from build123d import *

# Parameters (mm, degrees)
SKETCH1_W            = 604
SKETCH1_H            = 470
BOSS_EXTRUDE1_DEPTH  = 3
FILLET1_R            = 3
M5_CLEARANCE_HOLE1_D = 5.5
CUT_EXTRUDE5_DEPTH   = 766.326727614
SKETCH10_W           = 50
SKETCH10_H           = 80
CUT_EXTRUDE6_DEPTH   = 766.326727614
FILLET5_R            = 3


with BuildPart() as part:
    # Sketch1 → Boss-Extrude1 (new body)
    with BuildSketch(Plane.XY):
        with Locations((302, 235)):
            Rectangle(SKETCH1_W, SKETCH1_H)
    extrude(amount=BOSS_EXTRUDE1_DEPTH)

    # Fillet1
    fillet1_edges = [part.edges().sort_by_distance(p)[0] for p in [
        (0, 470, 1.5),
        (604, 470, 1.5),
        (604, 0, 1.5),
        (0, 0, 1.5),
    ]]
    fillet(fillet1_edges, radius=FILLET1_R)

    # M5 Clearance Hole1 (through all)
    with Locations(Plane(origin=(0, 0, 0), x_dir=(-1, 0, 0), z_dir=(0, 0, -1))):
        with Locations((-594, 460), (-394, 460), (-210, 460), (-10, 460), (-10, 10), (-210, 10), (-394, 10), (-594, 10), (-544, 410), (-544, 60), (-35, 410), (-35, 60), (-109.625, 410), (-109.625, 60)):
            Hole(M5_CLEARANCE_HOLE1_D / 2)

    # Sketch9 → Cut-Extrude5 (cut, through all)
    with BuildSketch(Plane.XY.offset(3)):
        with BuildLine():
            Line((32, 412.75), (38, 412.75))
            ThreePointArc((38, 412.75), (40.75, 410), (38, 407.25))
            Line((38, 407.25), (32, 407.25))
            ThreePointArc((32, 407.25), (29.25, 410), (32, 412.75))
        make_face()
        with BuildLine():
            Line((106.625, 412.75), (112.625, 412.75))
            ThreePointArc((112.625, 412.75), (115.375, 410), (112.625, 407.25))
            Line((112.625, 407.25), (106.625, 407.25))
            ThreePointArc((106.625, 407.25), (103.875, 410), (106.625, 412.75))
        make_face()
        with BuildLine():
            Line((32, 62.75), (38, 62.75))
            ThreePointArc((38, 62.75), (40.75, 60), (38, 57.25))
            Line((38, 57.25), (32, 57.25))
            ThreePointArc((32, 57.25), (29.25, 60), (32, 62.75))
        make_face()
        with BuildLine():
            Line((106.625, 62.75), (112.625, 62.75))
            ThreePointArc((112.625, 62.75), (115.375, 60), (112.625, 57.25))
            Line((112.625, 57.25), (106.625, 57.25))
            ThreePointArc((106.625, 57.25), (103.875, 60), (106.625, 62.75))
        make_face()
        with BuildLine():
            Line((541, 412.75), (547, 412.75))
            ThreePointArc((547, 412.75), (549.75, 410), (547, 407.25))
            Line((547, 407.25), (541, 407.25))
            ThreePointArc((541, 407.25), (538.25, 410), (541, 412.75))
        make_face()
        with BuildLine():
            Line((541, 62.75), (547, 62.75))
            ThreePointArc((547, 62.75), (549.75, 60), (547, 57.25))
            Line((547, 57.25), (541, 57.25))
            ThreePointArc((541, 57.25), (538.25, 60), (541, 62.75))
        make_face()
    extrude(amount=-CUT_EXTRUDE5_DEPTH, mode=Mode.SUBTRACT)

    # Sketch10 → Cut-Extrude6 (cut, through all)
    with BuildSketch(Plane.XY.offset(3)):
        with Locations((579, 60)):
            Rectangle(SKETCH10_W, SKETCH10_H)
    extrude(amount=-CUT_EXTRUDE6_DEPTH, mode=Mode.SUBTRACT)

    # Fillet5
    fillet5_edges = [part.edges().sort_by_distance(p)[0] for p in [
        (604, 100, 1.5),
        (604, 20, 1.5),
    ]]
    fillet(fillet5_edges, radius=FILLET5_R)


solid = part.part
Input: part model. Units: mm. Frame: model coordinates. Round coordinates to 2 decimals unless told otherwise and drop trailing zeros. Write each loop counter-clockwise with the first axis right and the second up, starting at its lowest first coordinate (ties: lowest second). Pieces come first, ordered by that corner, then holes.
1) Cut plane A-A (y = 85). Return the cut outline in (x, z).
2) Cut plane B-B (z = 1.3). Count the separate pieces of the cut face and the enclosed holes in it, then the cut area to 3 significant figures.
3) Ray query, L1, parallel to Y at x = 10, z = 0.9; L2, parallel to X at y = 460, z = 1.8; L3, parallel to X at y = 92, z = 1.8. Return the intervals inside material, ascending.
Geometry says:
1. outline: (0, 0) - (554, 0) - (554, 3) - (0, 3) - close
2. separate pieces: 1
2. enclosed holes: 14
2. area: 279,000 mm2
3. L1: y = 0 to 7.25, 12.75 to 457.25, 462.75 to 470
3. L2: x = 0 to 7.25, 12.75 to 207.25, 212.75 to 391.25, 396.75 to 591.25, 596.75 to 604
3. L3: x = 0 to 554
